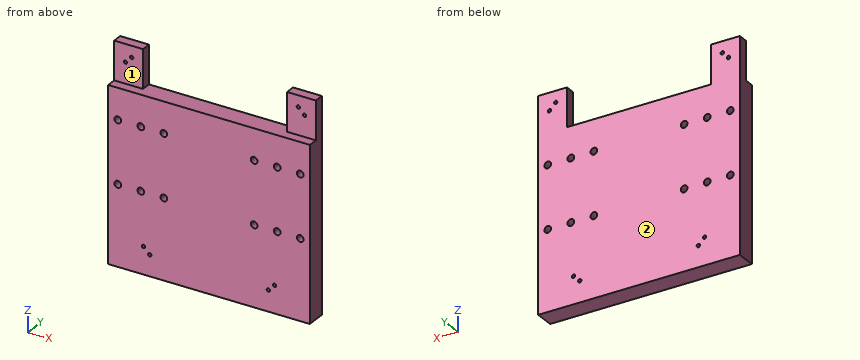
Autodesk Inventor part; units mm, degrees
ref_plane "YZ Plane" through (0, 0, 0) normal (1, 0, 0) x (0, 1, 0)
ref_plane "XZ Plane" through (0, 0, 0) normal (0, 1, 0) x (-1, 0, 0)
ref_plane "XY Plane" through (0, 0, 0) normal (0, 0, 1) x (1, 0, 0)
sketch "Boceto1" plane through (0, 0, 0) normal (0, 1, 0) x (-1, 0, 0)
  line L0 (105, 90) -> (-105, 90)
  line L1 (-105, 90) -> (-105, -90)
  line L2 (-105, -90) -> (105, -90)
  line L3 (105, -90) -> (105, 90)
  line L4 (105, 90) -> (-105, -90) construction
  line L5 (-105, 90) -> (105, -90) construction
  point P0 (0, 0)
  dimension "d0" = 210
  dimension "d1" = 180
extrude "Extrusión1" add sketch "Boceto1" along normal blind 20
sketch "Boceto2" plane through (0, 20, 0) normal (0, 1, 0) x (1, 0, 0)
  circle A0 centre (-95, -57.83) radius 3.5
  line L0 (-105, -65.43) -> (-37, -65.43)
  line L1 (-37, -65.43) -> (-37, 14.57)
  line L2 (-37, 14.57) -> (-105, 14.57)
  line L3 (-105, 14.57) -> (-105, -65.43)
  line L4 (-71, -65.43) -> (-71, -8.508)
  circle A1 centre (-71, -57.83) radius 3.5
  circle A2 centre (-47, -57.83) radius 3.5
  line L5 (-37, -25.43) -> (-48.2072, -25.43)
  circle A3 centre (-47, 6.97) radius 3.5
  circle A4 centre (-71, 6.97) radius 3.5
  circle A5 centre (-95, 6.97) radius 3.5
  line L6 (0, 0) -> (0, 47.1145)
  circle A6 centre (95, -57.83) radius 3.5
  line L7 (105, -65.43) -> (37, -65.43)
  line L8 (37, -65.43) -> (37, 14.57)
  line L9 (37, 14.57) -> (105, 14.57)
  line L10 (105, 14.57) -> (105, -65.43)
  line L11 (71, -65.43) -> (71, -8.508)
  circle A7 centre (71, -57.83) radius 3.5
  circle A8 centre (47, -57.83) radius 3.5
  line L12 (37, -25.43) -> (48.2072, -25.43)
  circle A9 centre (47, 6.97) radius 3.5
  circle A10 centre (71, 6.97) radius 3.5
  circle A11 centre (95, 6.97) radius 3.5
  circle A12 centre (-65, 65) radius 5
  circle A13 centre (65, 65) radius 5
  circle A14 centre (65, 65) radius 5
  line L13 (0, 0) -> (210, 0)
  line L14 (0, 0) -> (210, 0)
  line L15 (210, 0) -> (105, 0)
  circle A15 centre (40, -25) radius 5
  circle A16 centre (0, -75) radius 10
  line L16 (-105, -90) -> (105, -90)
  line L17 (105, 90) -> (-105, 90)
  line L18 (-105, 90) -> (-105, -90)
  dimension "d4" = 7
  dimension "d5" = 68
  dimension "d6" = 80
  dimension "d7" = 7.6
  dimension "d8" = 10
  dimension "d9" = 7
  dimension "d11" = 24
  dimension "d14" = 10
  dimension "d16" = 10
  dimension "d30" = 20
  dimension "d31" = 0
  dimension "d32" = 15
  dimension "d101" = 25
  dimension "d102" = 40
extrude "Extrusión2" cut sketch "Boceto2" against normal blind 20 contours A0 | A1 L4 | L4 A1 | A2 | A3 | A4 | A5 | A6 | A7 L11 | L11 A7 | A8 | A9 | A10 | A11
sketch "Boceto7" plane through (-105, 0, 90) normal (0, 0, 1) x (1, 0, 0)
  line L0 (0, 10) -> (29.9999, 10)
  line L1 (29.9999, 20) -> (29.9999, 10)
  line L2 (0, 10) -> (29.9999, 10)
  line L3 (29.9999, 10) -> (29.9999, 20)
  line L4 (29.9999, 20) -> (0, 20)
  line L5 (0, 20) -> (0, 10)
  line L6 (180.0001, 10) -> (210, 10)
  line L7 (210, 10) -> (210, 20)
  line L8 (180.0001, 10) -> (210, 10)
  line L9 (210, 10) -> (210, 20)
  line L10 (210, 20) -> (180.0001, 20)
  line L11 (180.0001, 20) -> (180.0001, 10)
  line L12 (0, 0) -> (0, 20)
  line L13 (210, 0) -> (210, 20)
  point P0 (105, 0)
  point P1 (0, 10)
  dimension "d79" = 29.9999
  dimension "d80" = 10
  dimension "d81" = 0
  dimension "d82" = 10
  dimension "d83" = 29.9999
  dimension "d84" = 0
extrude "Extrusión7" add sketch "Boceto7" along normal blind 40
sketch "Boceto8" plane through (0, 20, 0) normal (0, 1, 0) x (1, 0, 0)
  line L0 (-105, -90) -> (-105, -130)
  line L1 (-64.3507, -90) -> (-74.3507, -90)
  line L2 (-105, -130) -> (-75.0001, -130)
  line L3 (-75.0001, -130) -> (-75.0001, -90)
  line L4 (-75.0001, -90) -> (-105, -90)
  line L5 (-55.1959, -89.9497) -> (-75.0001, -90)
  circle A0 centre (-93.25, -111.75) radius 1.75
  circle A1 centre (-86.75, -118.25) radius 1.75
  line L6 (-75.0001, -90) -> (75.0001, -90)
  line L7 (0, -90) -> (0, -111.75)
  circle A2 centre (86.75, -118.25) radius 1.75
  circle A3 centre (93.25, -111.75) radius 1.75
  point P0 (0, 0)
  point P1 (-63.4459, -118.25)
  point P2 (-86.75, -111.75)
  point P3 (-105, -16)
  point P4 (86.75, -111.75)
  dimension "d67" = 11.7499
  dimension "d86" = 40
  dimension "d87" = 29.9999
  dimension "d88" = 21.75
  dimension "d89" = 11.75
  dimension "d90" = 28.3003
  dimension "d91" = 11.7499
hole "Agujero1" at (-86.75, 20, 118.25) at (-93.25, 20, 111.75) at (86.75, 20, 118.25) at (93.25, 20, 111.75) direction (0, -1, 0) diameter 3.5 end through all
sketch "Boceto9" plane through (0, 20, 0) normal (0, 1, 0) x (1, 0, 0)
  circle A0 centre (61.7786, 68.221) radius 1.75
  line L0 (60.0286, 59.971) -> (70.0286, 59.971)
  line L1 (70.0286, 59.971) -> (70.0286, 69.971)
  line L2 (70.0286, 69.971) -> (60.0286, 69.971)
  line L3 (60.0286, 69.971) -> (60.0286, 59.971)
  line L4 (60.0286, 59.971) -> (70.0286, 69.971) construction
  line L5 (70.0286, 59.971) -> (60.0286, 69.971) construction
  circle A1 centre (68.2786, 61.721) radius 1.75
  line L6 (105, 90) -> (-105, 90)
  line L7 (-60.0286, 69.971) -> (-60.0286, 59.971)
  line L8 (-70.0286, 59.971) -> (-70.0286, 69.971)
  line L9 (-60.0286, 59.971) -> (-70.0286, 69.971) construction
  line L10 (-70.0286, 59.971) -> (-60.0286, 69.971) construction
  line L11 (-60.0286, 59.971) -> (-70.0286, 59.971)
  circle A2 centre (-68.2786, 61.721) radius 1.75
  line L12 (-70.0286, 69.971) -> (-60.0286, 69.971)
  circle A3 centre (-61.7786, 68.221) radius 1.75
  point P0 (0, 0)
  point P1 (70.0286, 64.971)
  point P2 (-70.0286, 64.971)
extrude "Extrusión8" cut sketch "Boceto9" against normal blind 20 contours A0 | A1 | A3 | A2
properties part number "base_back"
Verification items for the finished model (mm, model axes). Face numbers are marked on the shaded views. A direction names the side the tool comes from. Coordinates: 2 decimals unless noted, no trailing zeros. Write each loop counter-clockwise with the first axis right and the second up, starting at its lowest first coordinate (ties: lowest second). Pieces come first, ordered by that corner, then holes. Notation, with made-up numbers: (51.5, -34.5) - (103.5, -34.5) arc R18 cw to (103.5, -5.5) - close; hole circle Ø2 at (-33.5, -5). An arc over 180 degrees is marked (long way). Answer as a JSON object with one key per item and string values.
(1) Tool access check on the marked faces 1 and 2. Record the directions out of +Z, -Z, +X, -X, +Y, -Y that give a thin tool (end or side, any length) a straight path to the whole face; none if there is none.
Report:
{"face 1": "+Z, +X, -X, -Y", "face 2": "+Z, -Z, +X, -X, +Y"}
(2) Cross-section at B-B on y = 15.75. Give the number of separate pieces and of enclosed holes in the cut face, plus the area to 3 significant figures.
Report:
{"separate pieces": "1", "enclosed holes": "20", "area": "39,700 mm^2"}
(3) Thickness scan on line 1 along Z through (x, y) = (95, 5.25); line 2 along X through (y, z) = (3, -61); line 3 along X through (y, z) = (13, 99.5). Record the ranges inside material, lowest first.
Report:
{"line 1": "-90 to -10.47, -3.47 to 54.33, 61.33 to 90", "line 2": "-105 to -69.87, -66.68 to 66.68, 69.87 to 105", "line 3": "-105 to -75, 75 to 105"}
(4) Gauge pin test, flat ends, axial feed: pin 1 Ø11 at (x, z) = (71, -6.97) entering from +Y; pin 2 Ø5.5 at (x, z) = (-93.25, 111.75) entering from -Y. Record the tip position at first contact, or that the pin passes through.
Report:
{"pin 1": "y = 20", "pin 2": "y = 10"}
(5) Cross-section at A-A on z = 57.83. Record the cut outline in (x, y), plus the area to 3 significant figures.
Report:
{"outline": "(-105, 0) - (-98.5, 0) - (-98.5, 20) - (-105, 20) - close; (-91.5, 0) - (-74.5, 0) - (-74.5, 20) - (-91.5, 20) - close; (-67.5, 0) - (-50.5, 0) - (-50.5, 20) - (-67.5, 20) - close; (-43.5, 0) - (43.5, 0) - (43.5, 20) - (-43.5, 20) - close; (50.5, 0) - (67.5, 0) - (67.5, 20) - (50.5, 20) - close; (74.5, 0) - (91.5, 0) - (91.5, 20) - (74.5, 20) - close; (98.5, 0) - (105, 0) - (105, 20) - (98.5, 20) - close", "area": "3,360 mm^2"}
(6) Cross-section at C-C on x = 13.5. Record the cut outline in (y, z), plus the area to 3 significant figures.
Report:
{"outline": "(0, -90) - (20, -90) - (20, 90) - (0, 90) - close", "area": "3,600 mm^2"}
